Input: part model. Units: mm. Frame: model coordinates. A direction names the side the tool comes from. Round coordinates to 2 decimals unless told otherwise and drop trailing zeros. Loops run counter-clockwise (first coordinate to the right, second up) from the corner with the lowest first, then second, coordinate; pieces in that order, holes last. Notation, with made-up numbers: (14, 71.25) - (50, 71.25) arc R11 ccw to (50, 84.25) - close; hole circle Ø1 at (48, -36). An arc over 180 degrees is marked (long way). One line per question, with ' | ' between items. Start each with the question number.
Item 1: Section C-C, the plane x = 10. Return loops of the section in (y, z), plus the area to 3 significant figures.
Item 2: Section A-A, the plane y = -1.5. Return loops of the section in (x, z).
Item 3: Set-up query: faces 4 (the face through (17.5, 0, 1)), 5 (the face through (26.364, 14.476, 0.285)). Return all of +Z, -Z, +X, -X, +Y, -Y with unobstructed straight access to the full face (end or side cutting, diameter ignored); none if empty.
Item 4: Draft query along X for faces 1 (the face through (15, -33, 1)), 2 (the face through (-1, -13, 3)), 3 (the face through (27.897, -23.651, 1.493)). Return one class per face: pulls with the +X half, pulls with the -X half, needs draft (parallel to the pull), parting line crosses it, or undercut.
Item 5: Material intervals for line 1 along Y through (x, z) = (-13.5, 1.75); line 2 along Y through (x, z) = (-29, 0.3); line 3 along X through (y, z) = (17.5, 1.3), sorted ascending.
Item 6: Section B-B, the plane x = 1.5. Return loops of the section in (y, z), plus the area to 3 significant figures.
Item 7: First-contact query: pin 1 (3 mm diameter, centred on x = -28, y = 5, fed in from -Z). Flat tip, straight axial feed; report the tip coordinate or a pass-through.
Item 8: Section D-D, the plane x = 21. Give the number of separate pieces and of enclosed holes in the cut face, plus the area to 3 significant figures.
```python
from build123d import *

# Parameters (mm, degrees)
BOSS_EXTRUDE1_DEPTH = 3
SKETCH2_R           = 2.5
CUT_EXTRUDE1_DEPTH  = 10
CUT_EXTRUDE2_DEPTH  = 10
SKETCH5_R           = 2.5
CUT_EXTRUDE3_DEPTH  = 10
FILLET1_R           = 1


with BuildPart() as part:
    # Sketch1 → Boss-Extrude1 (new body)
    with BuildSketch(Plane.XY):
        Polygon((-13.5, 29), (-40, 0), (-40, -6), (-16, -41), (16, -41), (40, -6), (40, 0), (13.5, 29), align=None)
    extrude(amount=BOSS_EXTRUDE1_DEPTH)

    # Sketch2 → Cut-Extrude1 (cut)
    with BuildSketch(Plane(origin=(0, 0, 0), x_dir=(-1, 0, 0), z_dir=(0, 0, -1))):
        with Locations((-10, 19)):
            Circle(SKETCH2_R)
        with Locations((10, 19)):
            Circle(SKETCH2_R)
        with Locations((-13.5, -35)):
            Circle(SKETCH2_R)
        with Locations((13.5, -35)):
            Circle(SKETCH2_R)
    extrude(amount=-CUT_EXTRUDE1_DEPTH, mode=Mode.SUBTRACT)

    # Sketch3 → Cut-Extrude2 (cut)
    with BuildSketch(Plane(origin=(0, 0, 0), x_dir=(-1, 0, 0), z_dir=(0, 0, -1))):
        Polygon((24.5, 0), (24.5, 10.5), (-17.5, 10.5), (-17.5, -10.5), (24.5, -10.5), align=None)
    extrude(amount=-CUT_EXTRUDE2_DEPTH, mode=Mode.SUBTRACT)

    # Sketch5 → Cut-Extrude3 (cut)
    with BuildSketch(Plane.XY.offset(3)):
        with Locations((-28, -5)):
            Circle(SKETCH5_R)
        with Locations((-28, 5)):
            Circle(SKETCH5_R)
        with Locations((22, -5)):
            Circle(SKETCH5_R)
        with Locations((22, 5)):
            Circle(SKETCH5_R)
    extrude(amount=-CUT_EXTRUDE3_DEPTH, mode=Mode.SUBTRACT)

    # Fillet1
    fillet1_edges = [part.edges().sort_by_distance(p)[0] for p in [
        (-40, -3, 3),
        (-26.75, 14.5, 0),
        (0, 29, 0),
        (-28, -23.5, 3),
        (13.5, 29, 1.5),
        (40, 0, 1.5),
        (40, -6, 1.5),
        (16, -41, 1.5),
        (-16, -41, 1.5),
        (-40, -6, 1.5),
        (-40, 0, 1.5),
        (-13.5, 29, 1.5),
        (0, -41, 3),
        (28, -23.5, 3),
        (40, -3, 3),
        (26.75, 14.5, 3),
        (0, 29, 3),
        (-26.75, 14.5, 3),
        (26.75, 14.5, 0),
        (40, -3, 0),
        (28, -23.5, 0),
        (0, -41, 0),
        (-28, -23.5, 0),
        (-40, -3, 0),
    ]]
    fillet(fillet1_edges, radius=FILLET1_R)


solid = part.part
```
Return value:
1) outline: (-41, 1) arc R1 ccw to (-40, 0) - (-10.5, 0) - (-10.5, 3) - (-40, 3) arc R1 ccw to (-41, 2) - close; (10.5, 0) - (16.5, 0) - (16.5, 3) - (10.5, 3) - close; (21.5, 0) - (28, 0) arc R1 ccw to (29, 1) - (29, 2) arc R1 ccw to (28, 3) - (21.5, 3) - close | area: 131 mm2
2) outline: (-40, 1) arc R1 ccw to (-39, 0) - (-24.5, 0) - (-24.5, 3) - (-39, 3) arc R1 ccw to (-40, 2) - close; (17.5, 0) - (39, 0) arc R1 ccw to (40, 1) - (40, 2) arc R1 ccw to (39, 3) - (17.5, 3) - close
3) face 4: +Z, -Z | face 5: -Z, +X, +Y
4) face 1: undercut | face 2: needs draft | face 3: pulls with the +X half
5) line 1: -41 to -37.5, -32.5 to -10.5, 10.5 to 28.9 | line 2: -21.54 to -7.29, -2.71 to 2.71, 7.29 to 11.61 | line 3: -24.01 to -12, -8 to 8, 12 to 24.01
6) outline: (-41, 1) arc R1 ccw to (-40, 0) - (-10.5, 0) - (-10.5, 3) - (-40, 3) arc R1 ccw to (-41, 2) - close; (10.5, 0) - (28, 0) arc R1 ccw to (29, 1) - (29, 2) arc R1 ccw to (28, 3) - (10.5, 3) - close | area: 146 mm2
7) pin 1: through
8) separate pieces: 3 | enclosed holes: 0 | area: 135 mm2
